Part model, mm, in its own coordinate system. Round coordinates to 2 decimals unless told otherwise and drop trailing zeros. Write each loop counter-clockwise with the first axis right and the second up, starting at its lowest first coordinate (ties: lowest second). Pieces come first, ordered by that corner, then holes.
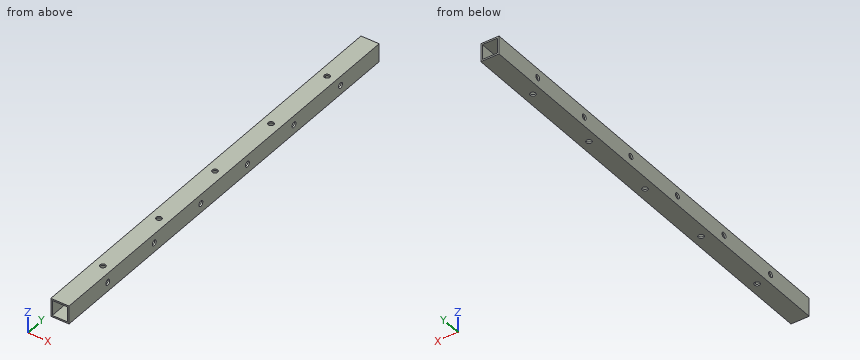
```python
from build123d import *

# Parameters (mm, degrees)
SKETCH1_W                 = 19.05
SKETCH1_H                 = 19.05
SKETCH1_W_2               = 15.875
SKETCH1_H_2               = 15.875
TUBE_DEPTH                = 457.753199808
SKETCH2_R                 = 2.8956
TOPPLATEHOLES_DEPTH       = 459.24842614
LPATTERN1_COUNT           = 5
LPATTERN1_PITCH           = 82.739099952
SKETCH3_R                 = 2.8956
SIDEPLATEHOLEMASTER_DEPTH = 459.24842614
LPATTERN2_COUNT           = 6
LPATTERN2_PITCH           = 68.690639962


with BuildPart() as part:
    # Sketch1 → Tube (new body)
    with BuildSketch(Plane(origin=(0, 0, 0), x_dir=(1, 0, 0), z_dir=(0, 1, 0))):
        Rectangle(SKETCH1_W, SKETCH1_H)
        Rectangle(SKETCH1_W_2, SKETCH1_H_2, mode=Mode.SUBTRACT)
    extrude(amount=TUBE_DEPTH)

    # Sketch2 → TopPlateHoles (cut, through all)
    with BuildSketch(Plane.XY.offset(9.525)):
        with Locations((0, 394.354799808)):
            Circle(SKETCH2_R)
    topplateholes = extrude(amount=-TOPPLATEHOLES_DEPTH, mode=Mode.SUBTRACT)

    # LPattern1: TopPlateHoles ×5
    with Locations(*[(0, -i * LPATTERN1_PITCH, 0) for i in range(1, LPATTERN1_COUNT)]):
        add(topplateholes, mode=Mode.SUBTRACT)

    # Sketch3 → SidePlateHoleMaster (cut, through all)
    with BuildSketch(Plane.ZY.offset(9.525)):
        with Locations((0, 400.603199808)):
            Circle(SKETCH3_R)
    sideplateholemaster = extrude(amount=-SIDEPLATEHOLEMASTER_DEPTH, mode=Mode.SUBTRACT)

    # LPattern2: SidePlateHoleMaster ×6
    with Locations(*[(0, -i * LPATTERN2_PITCH, 0) for i in range(1, LPATTERN2_COUNT)]):
        add(sideplateholemaster, mode=Mode.SUBTRACT)


solid = part.part
```
Q1. Wall check: L1, parallel to X at y = 162, z = -3.25 (1 decimal). Give the ranges that are in metal, low to high.
Values follow:
L1: x = -9.5 to -7.9, 7.9 to 9.5
Q2. Cut at B-B on x = 0. State how many separate pieces and enclosed holes the cut face has, plus the area to 3 significant figures.
Values follow:
separate pieces: 12
enclosed holes: 0
area: 1,360 mm2
Q3. Cut at A-A on y = 239. Write the cut outline in (x, z) (1 decimal).
Values follow:
outline: (-9.5, -9.5) - (9.5, -9.5) - (9.5, 9.5) - (-9.5, 9.5) - close; hole (-7.9, -7.9) - (7.9, -7.9) - (7.9, 7.9) - (-7.9, 7.9) - close
